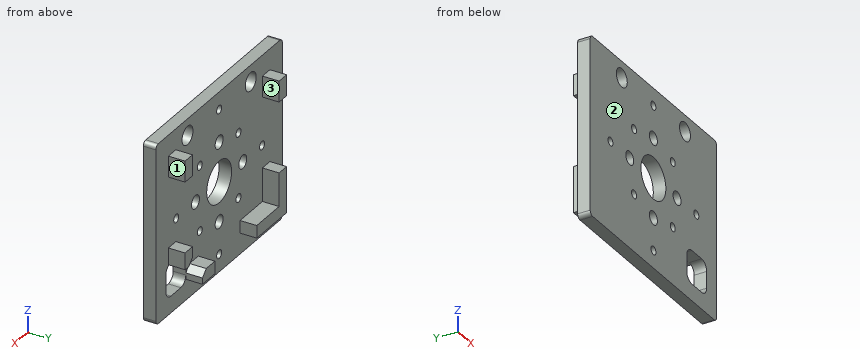
```python
from build123d import *

# Parameters (mm, degrees)
F0_W     = 50.8
F0_H     = 42.9
F0_R     = 1
F0_R_2   = 1.6
F0_R_3   = 5
F0_R_4   = 2.2
F1_DEPTH = 3
F2_R     = 1
F3_W     = 3
F3_H     = 5
F3_H_2   = 4
F3_W_2   = 5
F3_H_3   = 3
F4_DEPTH = 4
F5_SIZE  = 1.5


with BuildPart() as f1:
    # F0 (on Front) → F1 (new body)
    with BuildSketch(Plane.XZ):
        Rectangle(F0_W, F0_H)
        with Locations((0, -17.25)):
            Circle(F0_R, mode=Mode.SUBTRACT)
        with Locations((-7.7781745931, -7.7781745931)):
            Circle(F0_R, mode=Mode.SUBTRACT)
        with Locations((0, -9.5)):
            Circle(F0_R_2, mode=Mode.SUBTRACT)
        with BuildLine():
            ThreePointArc((21.4, -15.45), (20.8142135624, -16.8642135624), (19.4, -17.45))
            Line((19.4, -17.45), (15.4, -17.45))
            ThreePointArc((15.4, -17.45), (13.9857864376, -16.8642135624), (13.4, -15.45))
            Line((13.4, -15.45), (13.4, -11.45))
            ThreePointArc((13.4, -11.45), (13.9857864376, -10.0357864376), (15.4, -9.45))
            Line((15.4, -9.45), (19.4, -9.45))
            ThreePointArc((19.4, -9.45), (20.8142135624, -10.0357864376), (21.4, -11.45))
            Line((21.4, -11.45), (21.4, -15.45))
        make_face(mode=Mode.SUBTRACT)
        with Locations((7.7781745931, -7.7781745931)):
            Circle(F0_R, mode=Mode.SUBTRACT)
        with Locations((-17.25, 0)):
            Circle(F0_R, mode=Mode.SUBTRACT)
        with Locations((-9.5, 0)):
            Circle(F0_R_2, mode=Mode.SUBTRACT)
        Circle(F0_R_3, mode=Mode.SUBTRACT)
        with Locations((-7.7781745931, 7.7781745931)):
            Circle(F0_R, mode=Mode.SUBTRACT)
        with Locations((0, 9.5)):
            Circle(F0_R_2, mode=Mode.SUBTRACT)
        with Locations((-12.7, 17.5)):
            Circle(F0_R_4, mode=Mode.SUBTRACT)
        with Locations((0, 17.25)):
            Circle(F0_R, mode=Mode.SUBTRACT)
        with Locations((9.5, 0)):
            Circle(F0_R_2, mode=Mode.SUBTRACT)
        with Locations((7.7781745931, 7.7781745931)):
            Circle(F0_R, mode=Mode.SUBTRACT)
        with Locations((17.25, 0)):
            Circle(F0_R, mode=Mode.SUBTRACT)
        with Locations((12.7, 17.5)):
            Circle(F0_R_4, mode=Mode.SUBTRACT)
    extrude(amount=F1_DEPTH)

    # F2
    f2_edges = [f1.edges().sort_by_distance(p)[0] for p in [
        (25.4, -1.5, 21.45),
        (25.4, -1.5, -21.45),
        (-25.4, -1.5, -21.45),
        (-25.4, -1.5, 21.45),
    ]]
    fillet(f2_edges, radius=F2_R)

    # F3 (on face) → F4 (join)
    with BuildSketch(Plane(origin=(0, 0, 0), x_dir=(-1, 0, 0), z_dir=(0, 1, 0))):
        with Locations((-18.9, 13.95)):
            Rectangle(F3_W, F3_H)
        with Locations((-18.9, -7.45)):
            Rectangle(F3_W, F3_H_2)
        with Locations((18.9, 13.95)):
            Rectangle(F3_W, F3_H)
        Polygon((20.4, -16.45), (20.4, -5.45), (17.4, -5.45), (17.4, -13.45), (8.4, -13.45), (8.4, -16.45), align=None)
        with Locations((-10.9, -14.95)):
            Rectangle(F3_W_2, F3_H_3)
    extrude(amount=F4_DEPTH)

    # F5
    f5_edges = [f1.edges().sort_by_distance(p)[0] for p in [
        (13.4, 2, -13.45),
        (17.4, 2, -9.45),
    ]]
    chamfer(f5_edges, length=F5_SIZE)


solid = f1.part
```
Can you work these out from the model? Positions are in its coordinate system, mm. Face numbers are marked on the shaded views. Coordinates: 2 decimals unless noted, no trailing zeros. Loops run counter-clockwise (first coordinate to the right, second up) from the corner with the lowest first, then second, coordinate; pieces in that order, holes last.
1) Imagine slicing it at D-D on x = 0. List the corners of the cut face in (y, z) for me, plus the area to 3 significant figures.
2) I need wall thicknesses on probe 1 along Z at (x, y) = (0, -1.7); probe 2 along Z at (x, y) = (17.25, -0.7); probe 3 along X at (y, z) = (-2.25, -12.5). Which ranges of each line are inside material? Lowest first, please.
3) Imagine slicing it at C-C on z = 0. List the corners of the cut face in (x, y) for me, plus the area to 3 significant figures.
4) Imagine slicing it at B-B on y = 1.5. List the corners of the cut face in (x, z) for me, plus the area to 3 significant figures.
5) For pin 1 (4 mm diameter, centred on x = 0, z = 9.5, fed in from +Y); pin 2 (3.5 mm diameter, centred on x = -19.5, y = 2, fed in from -Z); pin 3 (1.2 mm diameter, centred on y = 1, z = 13, fed in from -X), each with a flat end and sliding along its axis, tell me the tip position at first contact or that it passes through.
6) Imagine slicing it at A-A on x = 9.5. List the corners of the cut face in (y, z) for me.
7) Thinking about a two-plate mould opening in X: for the marked faces 1, 2 and 3, which applies, pulls with the +X half, pulls with the -X half, needs draft (parallel to the pull), parting line crosses it, or undercut?
Completed:
1. outline: (-3, -21.45) - (0, -21.45) - (0, -18.25) - (-3, -18.25) - close; (-3, -16.25) - (0, -16.25) - (0, -11.1) - (-3, -11.1) - close; (-3, -7.9) - (0, -7.9) - (0, -5) - (-3, -5) - close; (-3, 5) - (0, 5) - (0, 7.9) - (-3, 7.9) - close; (-3, 11.1) - (0, 11.1) - (0, 16.25) - (-3, 16.25) - close; (-3, 18.25) - (0, 18.25) - (0, 21.45) - (-3, 21.45) - close
1. area: 67.5 mm2
2. probe 1: z = -21.45 to -18.25, -16.25 to -11.1, -7.9 to -5, 5 to 7.9, 11.1 to 16.25, 18.25 to 21.45
2. probe 2: z = -21.45 to -17.45, -9.45 to -1, 1 to 21.45
2. probe 3: x = -25.4 to 13.4, 21.4 to 25.4
3. outline: (-25.4, -3) - (-18.25, -3) - (-18.25, 0) - (-25.4, 0) - close; (-16.25, -3) - (-11.1, -3) - (-11.1, 0) - (-16.25, 0) - close; (-7.9, -3) - (-5, -3) - (-5, 0) - (-7.9, 0) - close; (5, -3) - (7.9, -3) - (7.9, 0) - (5, 0) - close; (11.1, -3) - (16.25, -3) - (16.25, 0) - (11.1, 0) - close; (18.25, -3) - (25.4, -3) - (25.4, 0) - (18.25, 0) - close
3. area: 91.2 mm2
4. outline: (-20.4, -16.45) - (-8.4, -16.45) - (-8.4, -13.45) - (-17.4, -13.45) - (-17.4, -5.45) - (-20.4, -5.45) - close; (-20.4, 11.45) - (-17.4, 11.45) - (-17.4, 16.45) - (-20.4, 16.45) - close; (8.4, -16.45) - (13.4, -16.45) - (13.4, -14.95) - (11.9, -13.45) - (8.4, -13.45) - close; (17.4, -7.95) - (18.9, -9.45) - (20.4, -9.45) - (20.4, -5.45) - (17.4, -5.45) - close; (17.4, 11.45) - (20.4, 11.45) - (20.4, 16.45) - (17.4, 16.45) - close
4. area: 115 mm2
5. pin 1: stops at y = 0
5. pin 2: stops at z = -16.45
5. pin 3: stops at x = -20.4
6. outline: (-3, -21.45) - (0, -21.45) - (0, -16.45) - (4, -16.45) - (4, -13.45) - (0, -13.45) - (0, -1.6) - (-3, -1.6) - close; (-3, 1.6) - (0, 1.6) - (0, 21.45) - (-3, 21.45) - close
7. face 1: pulls with the +X half
7. face 2: needs draft
7. face 3: undercut
